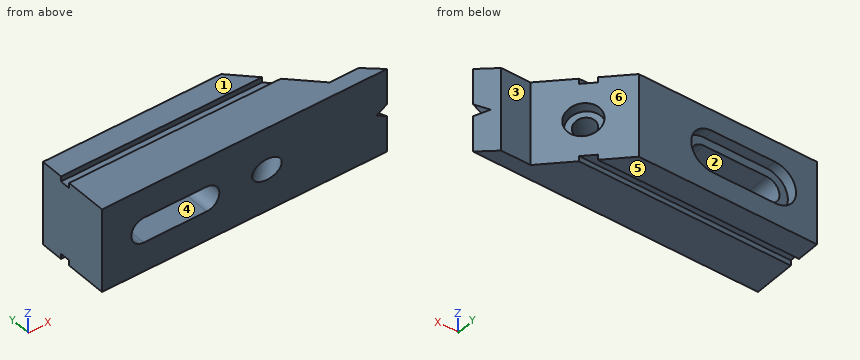
from build123d import *

# Parameters (mm, degrees)
BOSS_EXTRUDE1_DEPTH = 25.4
SKETCH2_R           = 6.35
CUT_EXTRUDE1_DEPTH  = 126.469958357
SKETCH3_R           = 10.16
CUT_EXTRUDE2_DEPTH  = 6.35
CUT_EXTRUDE3_DEPTH  = 179.420310783
SKETCH6_W           = 3.175
SKETCH6_H           = 6.35
CUT_EXTRUDE4_DEPTH  = 181.46516783
CUT_EXTRUDE5_DEPTH  = 6.35
CUT_EXTRUDE6_DEPTH  = 179.961882254


with BuildPart() as part:
    # Sketch1 → Boss-Extrude1 (new, symmetric)
    with BuildSketch(Plane.XY):
        Polygon((0, 0), (172.72, 0), (162.56, 8.89), (144.78, 8.89), (107.95, 45.72), (0, 45.72), align=None)
    extrude(amount=BOSS_EXTRUDE1_DEPTH, both=True)

    # Sketch2 → Cut-Extrude1 (cut, through all)
    with BuildSketch(Plane(origin=(76.835, 76.835, 0), x_dir=(0, 0, -1), z_dir=(0.7071067811865482, 0.7071067811865468, 0))):
        with Locations(Location((0, -70.688740495, 0), (0, 0, 90))):
            Circle(SKETCH2_R)
    extrude(amount=-CUT_EXTRUDE1_DEPTH, mode=Mode.SUBTRACT)

    # Sketch3 → Cut-Extrude2 (cut)
    with BuildSketch(Plane(origin=(76.835, 76.835, 0), x_dir=(0, 0, -1), z_dir=(0.7071067811865482, 0.7071067811865468, 0))):
        with Locations(Location((0, -70.688740495, 0), (0, 0, 90))):
            Circle(SKETCH3_R)
    extrude(amount=-CUT_EXTRUDE2_DEPTH, mode=Mode.SUBTRACT)

    # Sketch5 → Cut-Extrude3 (cut, through all)
    with BuildSketch(Plane(origin=(0, 8.89, 0), x_dir=(1, 0, 0), z_dir=(0, 1, 0))):
        Polygon((166.37, 0), (177.602369567, 6.485011593), (177.602369567, -6.485011593), align=None)
    extrude(amount=-CUT_EXTRUDE3_DEPTH, mode=Mode.SUBTRACT)

    # Sketch6 → Cut-Extrude4 (cut, through all)
    with BuildSketch(Plane(origin=(0, 0, 0), x_dir=(0, 0, -1), z_dir=(1, 0, 0))):
        with Locations((-23.8125, 28.575)):
            Rectangle(SKETCH6_W, SKETCH6_H)
        with Locations((23.8125, 28.575)):
            Rectangle(SKETCH6_W, SKETCH6_H)
    extrude(amount=CUT_EXTRUDE4_DEPTH, mode=Mode.SUBTRACT)

    # Sketch7 → Cut-Extrude5 (cut)
    with BuildSketch(Plane(origin=(0, 45.72, 0), x_dir=(1, 0, 0), z_dir=(0, 1, 0))):
        with BuildLine():
            Line((25.4, 12.7), (63.5, 12.7))
            ThreePointArc((63.5, 12.7), (76.2, 0), (63.5, -12.7))
            Line((63.5, -12.7), (25.4, -12.7))
            ThreePointArc((25.4, -12.7), (12.7, 0), (25.4, 12.7))
        make_face()
    extrude(amount=-CUT_EXTRUDE5_DEPTH, mode=Mode.SUBTRACT)

    # Sketch8 → Cut-Extrude6 (cut, through all)
    with BuildSketch(Plane(origin=(0, 39.37, 0), x_dir=(1, 0, 0), z_dir=(0, 1, 0))):
        with BuildLine():
            Line((25.4, -7.62), (63.5, -7.62))
            ThreePointArc((63.5, -7.62), (71.12, 0), (63.5, 7.62))
            Line((63.5, 7.62), (25.4, 7.62))
            ThreePointArc((25.4, 7.62), (17.78, 0), (25.4, -7.62))
        make_face()
    extrude(amount=-CUT_EXTRUDE6_DEPTH, mode=Mode.SUBTRACT)


solid = part.part
The listing builds one solid part. Answer for the finished solid, in the listing's coordinates (mm). Face numbers are marked on the shaded views. A direction names the side the tool comes from. Coordinates: 2 decimals unless noted, no trailing zeros. Loops run counter-clockwise (first coordinate to the right, second up) from the corner with the lowest first, then second, coordinate; pieces in that order, holes last. Notation, with made-up numbers: M -8,47 L 27,47 A22 ccw 27,73 Z; hole C 38.25,-3 d3. An arc over 180 degrees is marked long. Answer in a Markdown table with one row per item.
1) Which of the six approach directions +Z, -Z, +X, -X, +Y, -Y give full straight-line access (tool end or side, diameter ignored) to the marked faces 1, 2 and 3?
Answers below:
| item | result |
|---|---|
| face 1 | +Z, +X, -X, +Y, -Y |
| face 2 | +Y, -Y |
| face 3 | +Z, -Z, +X, +Y |
2) Given pin 1 (3 mm diameter, centred on x = 129, z = -4.5, fed in from +Y); pin 2 (1.9 mm diameter, centred on x = 41.5, y = 28, fed in from +Z) (3 decimals); pin 3 (19.5 mm diameter, centred on x = 149.5, z = 9, fed in from +Y), each flat-ended and moving along its own axis, determine where each tip first touches the part or whether it passes through.
Answers below:
| item | result |
|---|---|
| pin 1 | y = 18.07 |
| pin 2 | z = 22.225 |
| pin 3 | y = 13.92 |
3) Find section B-B (z = -18). Determine the outline of the cut face in (x, y), then the cut area to 3 significant figures.
Answers below:
| item | result |
|---|---|
| outline | M 0,0 L 172.72,0 L 162.56,8.89 L 144.78,8.89 L 107.95,45.72 L 0,45.72 Z |
| area | 6,140 mm^2 |
4) Determine the mould class of the marked faces 4, 5 and 6 for opening direction X: released by +X, released by -X, zero draft, split by the parting line, or undercut.
Answers below:
| item | result |
|---|---|
| face 4 | undercut |
| face 5 | zero draft |
| face 6 | released by +X |
5) Find the intervals of material crossed by probe 1 along Z at (x, y) = (33, 16.5); probe 2 along X at (y, z) = (8.5, 0.5); probe 3 along Z at (x, y) = (82.5, 27) (3 decimals), in increasing order.
Answers below:
| item | result |
|---|---|
| probe 1 | -25.4 to -7.62, 7.62 to 25.4 |
| probe 2 | 0 to 17.8, 71.1 to 99.52, 117.42 to 163.01 |
| probe 3 | -22.225 to 22.225 |
6) Find section A-A (x = 48.5). Determine the outline of the cut face in (y, z) (3 decimals), then the cut area to 3 significant figures.
Answers below:
| item | result |
|---|---|
| outline | M 0,-25.4 L 25.4,-25.4 L 25.4,-22.225 L 31.75,-22.225 L 31.75,-25.4 L 45.72,-25.4 L 45.72,-12.7 L 39.37,-12.7 L 39.37,-7.62 L 0,-7.62 Z; M 0,7.62 L 39.37,7.62 L 39.37,12.7 L 45.72,12.7 L 45.72,25.4 L 31.75,25.4 L 31.75,22.225 L 25.4,22.225 L 25.4,25.4 L 0,25.4 Z |
| area | 1,520 mm^2 |
7) Find section C-C (y = 4). Count the separate pieces of the cut face and the enclosed holes in it, then the cut area to 3 significant figures.
Answers below:
| item | result |
|---|---|
| separate pieces | 1 |
| enclosed holes | 2 |
| area | 7,600 mm^2 |
